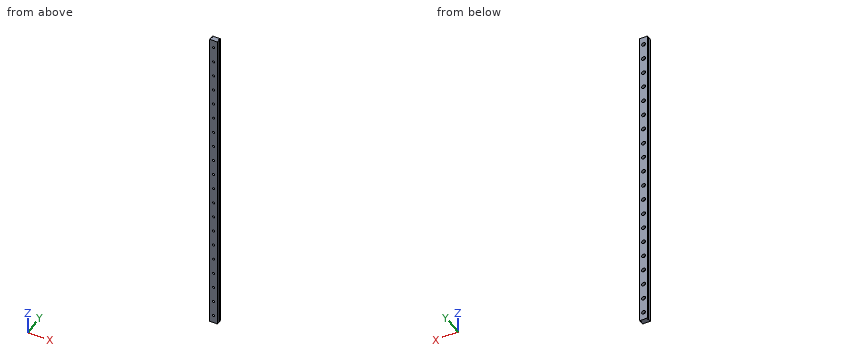
```python
from build123d import *

# Parameters (mm, degrees)
PAD073_DEPTH        = 500
HOLE001_D           = 3.4
HOLE001_CBORE_D     = 6.1
HOLE001_CBORE_DEPTH = 4.5
LINEARPATTERN_COUNT = 20
LINEARPATTERN_PITCH = 25


with BuildPart() as part:
    # Sketch119 → Pad073 (new body)
    with BuildSketch(Plane.XY):
        Polygon((-6, 0), (-6, 5), (-5, 5), (-5, 6), (-6, 6), (-6, 8), (6, 8), (6, 6), (5, 6), (5, 5), (6, 5), (6, 0), align=None)
    extrude(amount=PAD073_DEPTH)

    # Hole001 (through all)
    with Locations(Plane(origin=(0, 8, 0), x_dir=(1, 0, 0), z_dir=(0, 1, 0))):
        with Locations((0, -12.5)):
            hole001 = CounterBoreHole(HOLE001_D / 2, HOLE001_CBORE_D / 2, HOLE001_CBORE_DEPTH)

    # LinearPattern: Hole001 ×20
    with Locations(*[(0, 0, i * LINEARPATTERN_PITCH) for i in range(1, LINEARPATTERN_COUNT)]):
        add(hole001, mode=Mode.SUBTRACT)


solid = part.part
```
Input: part model. Units: mm. Frame: model coordinates. Give positions to 0.01 mm unless a question says otherwise; leave off trailing zeros.
1) Contact query for flat-ended pins moving along their axis: pin 1 (3.5 mm diameter, centred on x = 0, z = 37.5, fed in from +Y); pin 2 (5 mm diameter, centred on x = 2.5, z = 420.5, fed in from -Y). Output: stop coordinate, or through.
A:
pin 1: stops at y = 3.5
pin 2: stops at y = 0
2) Section query A-A on y = 1.25. Count the separate pieces of the cut face and the enclosed holes in it, and give its area (3 significant figures).
A:
separate pieces: 1
enclosed holes: 20
area: 5,820 mm2
3) Line query: L1, parallel to X at y = 2.75, z = 212.5; L2, parallel to X at y = 7.1, z = 87.5; L3, parallel to X at y = 5.5, z = 23. Output: solid intervals per line, ascending.
A:
L1: x = -6 to -1.7, 1.7 to 6
L2: x = -6 to -3.05, 3.05 to 6
L3: x = -5 to 5
